Work out the finished part from the listing and answer in its coordinate system (mm). Face numbers are marked on the shaded views. Give positions to 0.01 mm unless a question says otherwise; leave off trailing zeros. Loops run counter-clockwise (first coordinate to the right, second up) from the corner with the lowest first, then second, coordinate; pieces in that order, holes last. Notation, with made-up numbers: (83, -20.5) -> (102, -20.5) arc R27 cw to (102, -0.5) -> close; hole circle Ø7 at (54, 35.25). An arc over 180 degrees is marked (long way). Answer as CSV lines item,"result". Start each with the question number.
1. Find the intervals of material crossed by line 1 along Y through (x, z) = (-24, 11.75); line 2 along Z through (x, y) = (1.5, 7); line 3 along Z through (x, y) = (-17, -16.5), in increasing order.
2. Find section A-A, the plane x = 0. Give the vertices of the cut face in (y, z), and give its area (3 significant figures).
3. Find section D-D, the plane y = 22.5. Give the vertices of the cut face in (x, z), and give its area (3 significant figures).
4. Find section C-C, the plane z = -3. Give the vertices of the cut face in (x, y), and give its area (3 significant figures).
5. Flat-ended cylindrical pins translate along their axes: pin 1 Ø1 at (x, y) = (7, 26) entering from -Z; pin 2 Ø8 at (x, y) = (13, -23.5) entering from -Z; pin 3 Ø8 at (x, z) = (6, 16.5) entering from +Y; pin 4 Ø2 at (x, y) = (-25, 17) entering from -Z. Find the tip coordinate at first contact, or state that the pin passes through.
6. Determine the mould class of the marked faces 1, 2, 3 and 4 for opening direction Y: +Y half, -Y half, draft (parallel to the pull), parting line (faces both ways), or undercut.
7. Find section B-B, the plane y = -6.5. Give the vertices of the cut face in (x, z), and give its area (3 significant figures).
from build123d import *

# Parameters (mm, degrees)
F0_R     = 5
F1_DEPTH = 20
F2_DEPTH = 35
F4_R     = 8
F5_DEPTH = 3


with BuildPart() as f1:
    # F0 (on Front) → F1 (new body, symmetric)
    with BuildSketch(Plane.XZ):
        with BuildLine():
            Line((40, 20), (0, 20))
            Line((0, 20), (-40, 20))
            Line((-40, 20), (-40, 13.5))
            Line((-40, 13.5), (-4.9582247647, -6.5069341219))
            ThreePointArc((-4.9582247647, -6.5069341219), (0, -7.822695112), (4.9582247647, -6.5069341219))
            Line((4.9582247647, -6.5069341219), (40, 13.5))
            Line((40, 13.5), (40, 20))
        make_face()
        Circle(F0_R, mode=Mode.SUBTRACT)
    extrude(amount=F1_DEPTH, both=True)

    # F0 (on Front) → F2 (join, symmetric)
    with BuildSketch(Plane.XZ):
        Circle(F0_R)
    extrude(amount=F2_DEPTH, both=True)

    # F4 (on offset) → F5 (join)
    with BuildSketch(Plane.XZ.offset(27)):
        Circle(F4_R)
    extrude(amount=F5_DEPTH)

    # F6: F1 across plane


with BuildPart() as f1_1:
    add(f1.part)
    add(f1.part.mirror(Plane.XZ))


solid = f1_1.part
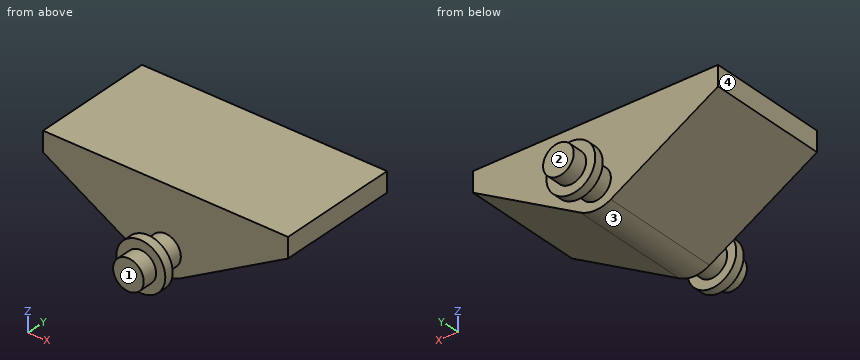
Resolved:
1,line 1,"y = -20 to 20"
1,line 2,"z = -7.71 to 20"
1,line 3,"z = 0.37 to 20"
2,outline,"(-35, -5) -> (-30, -5) -> (-30, -8) -> (-27, -8) -> (-27, -5) -> (-20, -5) -> (-20, -7.82) -> (20, -7.82) -> (20, -5) -> (27, -5) -> (27, -8) -> (30, -8) -> (30, -5) -> (35, -5) -> (35, 5) -> (30, 5) -> (30, 8) -> (27, 8) -> (27, 5) -> (20, 5) -> (20, 20) -> (-20, 20) -> (-20, 5) -> (-27, 5) -> (-27, 8) -> (-30, 8) -> (-30, 5) -> (-35, 5) -> close"
2,area,"1,450 mm^2"
3,outline,"circle Ø10 at (0, 0)"
3,area,"78.5 mm^2"
4,outline,"(-11.1, -20) -> (-4, -20) -> (-4, -27) -> (-7.42, -27) -> (-7.42, -30) -> (-4, -30) -> (-4, -35) -> (4, -35) -> (4, -30) -> (7.42, -30) -> (7.42, -27) -> (4, -27) -> (4, -20) -> (11.1, -20) -> (11.1, 20) -> (4, 20) -> (4, 27) -> (7.42, 27) -> (7.42, 30) -> (4, 30) -> (4, 35) -> (-4, 35) -> (-4, 30) -> (-7.42, 30) -> (-7.42, 27) -> (-4, 27) -> (-4, 20) -> (-11.1, 20) -> close"
4,area,"1,170 mm^2"
5,pin 1,"passes through"
5,pin 2,"stops at z = -3.02"
5,pin 3,"stops at y = 20"
5,pin 4,"stops at z = 4.36"
6,face 1,"-Y half"
6,face 2,"+Y half"
6,face 3,"undercut"
6,face 4,"draft"
7,outline,"(-40, 13.5) -> (-4.96, -6.51) arc R10 ccw to (4.96, -6.51) -> (40, 13.5) -> (40, 20) -> (-40, 20) -> close"
7,area,"1,430 mm^2"
